The model under review builds one solid part; all positions refer to its coordinate system, in mm. A direction names the side the tool comes from. Round coordinates to 2 decimals unless told otherwise and drop trailing zeros.
Item 1: Machinability: for faces 1 (the face through (0, -13, -296)), 2 (the face through (0, 4, 0)), which of the approach directions +Z, -Z, +X, -X, +Y, -Y give a long, thin tool a straight path to every point of the face, cutting with its end or side? Answer none if there is none.
Item 2: To check wall thickness, follow L1, parallel to Y at x = 0.25, z = -448; L2, parallel to X at y = 0, z = -246.5; L3, parallel to Y at x = 10, z = -222.5 (3 decimals). State the ranges of each line that lie inside material, in increasing order.
Item 3: Draft analysis for pull direction X (two halves, no side actions). For faces 3 (the face through (0, -15, -304)), 4 (the face through (13, 0, -304)), 5 (the face through (15, 0, -304)), state which applies: +X half, -X half, draft (parallel to the pull), parting line (faces both ways), or undercut.
Item 4: Add section A-A (z = -515). State how many separate pieces and enclosed holes the cut face has, plus the area to 3 significant figures.
Item 5: Clearance check with a flat-ended pin moving along its axis: pin 1 Ø2.5 at (x, y) = (-0.5, 9.5) entering from +Z. State where the tip first meets the part, or that it passes through.
Autodesk Inventor part; units mm, degrees
ref_plane "C1_XY" through (0, 0, 0) normal (0, 0, 1) x (1, 0, 0)
ref_plane "C1_YZ" through (0, 0, 0) normal (1, 0, 0) x (0, 1, 0)
ref_plane "C1_ZX" through (0, 0, 0) normal (0, 1, 0) x (0, 0, 1)
sketch "Sketch_122" plane through (0, 0, 0) normal (0, 0, 1) x (1, 0, 0)
  arc A0 (-15, -13) -> (-13, -15) centre (-13, -13) ccw
  line L0 (-13, -15) -> (13, -15)
  arc A1 (13, -15) -> (15, -13) centre (13, -13) ccw
  line L1 (15, -13) -> (15, 13)
  arc A2 (15, 13) -> (13, 15) centre (13, 13) ccw
  line L2 (13, 15) -> (-13, 15)
  arc A3 (-13, 15) -> (-15, 13) centre (-13, 13) ccw
  line L3 (-15, 13) -> (-15, 4)
  line L4 (-15, 4) -> (-13, 4)
  line L5 (-13, 4) -> (-13, 8.25)
  line L6 (-13, 8.25) -> (-9.6642, 8.25)
  line L7 (-9.6642, 8.25) -> (-6, 4.5858)
  line L8 (-6, 4.5858) -> (-6, 0.5196)
  line L9 (-6, 0.5196) -> (-5.7, 0)
  line L10 (-5.7, 0) -> (-6, -0.5196)
  line L11 (-6, -0.5196) -> (-6, -4.5858)
  line L12 (-6, -4.5858) -> (-9.6642, -8.25)
  line L13 (-9.6642, -8.25) -> (-13, -8.25)
  line L14 (-13, -8.25) -> (-13, -4)
  line L15 (-13, -4) -> (-15, -4)
  line L16 (-15, -4) -> (-15, -13)
  line L17 (6, -4.5858) -> (9.6642, -8.25)
  line L18 (9.6642, -8.25) -> (13, -8.25)
  line L19 (13, -8.25) -> (13, 8.25)
  line L20 (13, 8.25) -> (9.6642, 8.25)
  line L21 (9.6642, 8.25) -> (6, 4.5858)
  line L22 (6, 4.5858) -> (6, -4.5858)
extrude "Extrusion1" add sketch "Sketch_122" against normal blind 616
sketch "Sketch2" plane through (0, 0, -616) normal (0, 0, -1) x (-1, 0, 0)
  point P0 (0, 0)
hole "Hole1" at (0, 0, -616) direction (0, 0, 1) diameter 6.8 end through all
sketch "Sketch_173" plane through (0, 0, 0) normal (0, 0, 1) x (1, 0, 0)
  arc A0 (-9.8177, 12.6944) -> (-11.625, 9.525) centre (-11.625, 11.625) ccw
  line L0 (-11.625, 9.525) -> (-8.1108, 9.525)
  line L1 (-8.1108, 9.525) -> (-4.5858, 6)
  line L2 (-4.5858, 6) -> (4.5858, 6)
  line L3 (4.5858, 6) -> (8.1108, 9.525)
  line L4 (8.1108, 9.525) -> (11.625, 9.525)
  arc A1 (11.625, 9.525) -> (9.8177, 12.6944) centre (11.625, 11.625) ccw
  arc A2 (8.7013, 13) -> (9.8177, 12.6944) centre (9.3013, 13) ccw
  line L5 (8.7013, 13) -> (-8.7013, 13)
  arc A3 (-9.8177, 12.6944) -> (-8.7013, 13) centre (-9.3013, 13) ccw
extrude "Extrusion2" cut sketch "Sketch_173" against normal blind 600
sketch "Sketch_174" plane through (0, 0, 0) normal (0, 0, 1) x (1, 0, 0)
  arc A0 (-11.625, -9.525) -> (-9.8177, -12.6944) centre (-11.625, -11.625) ccw
  arc A1 (-8.7013, -13) -> (-9.8177, -12.6944) centre (-9.3013, -13) ccw
  line L0 (-8.7013, -13) -> (8.7013, -13)
  arc A2 (9.8177, -12.6944) -> (8.7013, -13) centre (9.3013, -13) ccw
  arc A3 (9.8177, -12.6944) -> (11.625, -9.525) centre (11.625, -11.625) ccw
  line L1 (11.625, -9.525) -> (8.1108, -9.525)
  line L2 (8.1108, -9.525) -> (4.5858, -6)
  line L3 (4.5858, -6) -> (-4.5858, -6)
  line L4 (-4.5858, -6) -> (-8.1108, -9.525)
  line L5 (-8.1108, -9.525) -> (-11.625, -9.525)
extrude "Extrusion3" cut sketch "Sketch_174" against normal blind 600
ref_plane "C1_XY" through (0, 0, 0) normal (0, 0, 1) x (1, 0, 0)
ref_plane "C1_YZ" through (0, 0, 0) normal (1, 0, 0) x (0, 1, 0)
ref_plane "C1_ZX" through (0, 0, 0) normal (0, 1, 0) x (0, 0, 1)
ref_plane "to_frame_cap1_XY" through (0, 0, 0) normal (0, 0, 1) x (1, 0, 0)
ref_plane "to_frame_cap1_YZ" through (0, 0, 0) normal (1, 0, 0) x (0, 1, 0)
ref_plane "to_frame_cap1_ZX" through (0, 0, 0) normal (0, 1, 0) x (0, 0, 1)
ref_plane "to_frame_cap2_XY" through (0, 0, -600) normal (0, 0, -1) x (1, 0, 0)
ref_plane "to_frame_cap2_YZ" through (0, 0, -600) normal (1, 0, 0) x (0, -1, 0)
ref_plane "to_frame_cap2_ZX" through (0, 0, -600) normal (0, -1, 0) x (0, 0, -1)
thread "Thread1"
thread "Thread2"
properties part number "HFSC6-3030-616" material "Aluminum 6061"
Numbers:
1. face 1: +Z
1. face 2: +Z, +X, -X, +Y, -Y
2. L1: y = -15 to -13, -6 to -3.39, 3.39 to 6, 13 to 15
2. L2: x = -5.7 to -3.4, 3.4 to 6, 13 to 15
2. L3: y = -15 to -12.955, -9.525 to -8.25, 8.25 to 9.525, 12.955 to 15
3. face 3: draft
3. face 4: undercut
3. face 5: +X half
4. separate pieces: 1
4. enclosed holes: 4
4. area: 360 mm2
5. pin 1: stops at z = -600
